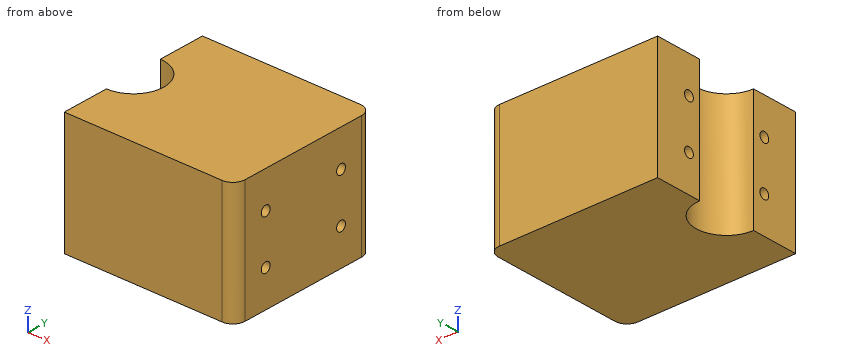
from build123d import *

# Parameters (mm, degrees)
F1_DEPTH = 25.4
F3_D     = 2.0828


# Not quite as in the source:
# - a feature names something its author has since deleted; it is built from what else it names


with BuildPart() as f1:
    # F0 (on Top) → F1 (new body)
    with BuildSketch(Plane.XY):
        with BuildLine():
            Line((-17.78, -6.35), (-17.78, -16.29156))
            Line((-17.78, -16.29156), (15.24, -16.29156))
            ThreePointArc((15.24, -16.29156), (17.0360512242, -15.5476112242), (17.78, -13.75156))
            Line((17.78, -13.75156), (17.78, 13.75156))
            ThreePointArc((17.78, 13.75156), (17.0360512242, 15.5476112242), (15.24, 16.29156))
            Line((15.24, 16.29156), (-17.78, 16.29156))
            Line((-17.78, 16.29156), (-17.78, 6.35))
            ThreePointArc((-17.78, 6.35), (-11.43, 0), (-17.78, -6.35))
        make_face()
    extrude(amount=F1_DEPTH)

    # F3 (through all)
    with Locations(Plane.YZ.offset(17.78)):
        with Locations((-8.89, 17.78), (-8.89, 7.62), (8.89, 17.78), (8.89, 7.62)):
            Hole(F3_D / 2)


solid = f1.part
Geometry: final body of the model. Coordinates: model frame, mm. Coordinates: 2 decimals unless noted, no trailing zeros. Write each loop counter-clockwise with the first axis right and the second up, starting at its lowest first coordinate (ties: lowest second). Pieces come first, ordered by that corner, then holes. Notation, with made-up numbers: (-6, -7.5) - (28, -7.5) arc R22 cw to (28, 27.5) - close; hole circle Ø9 at (32.25, -17). An arc over 180 degrees is marked (long way). Return JSON: item names as keys, results as strings.
Item 1: Section query D-D (z = 23.5). Output: boundary loops of the cut face in (x, y), and give its area (3 significant figures).
Completed:
{"outline": "(-17.78, -16.29) - (15.24, -16.29) arc R2.54 ccw to (17.78, -13.75) - (17.78, 13.75) arc R2.54 ccw to (15.24, 16.29) - (-17.78, 16.29) - (-17.78, 6.35) arc R6.35 cw to (-17.78, -6.35) - close", "area": "1,090 mm2"}
Item 2: Line query: L1, parallel to Z at x = -5, y = -8.89; L2, parallel to Z at x = 10, y = -8; L3, parallel to Y at x = -13.5, z = 4.25. Output: solid intervals per line, ascending.
Completed:
{"L1": "z = 0 to 6.58, 8.66 to 16.74, 18.82 to 25.4", "L2": "z = 0 to 7.08, 8.16 to 17.24, 18.32 to 25.4", "L3": "y = -16.29 to -4.69, 4.69 to 16.29"}
Item 3: Section query A-A (z = 7.62). Output: boundary loops of the cut face in (x, y), and give its area (3 significant figures).
Completed:
{"outline": "(-17.78, -16.29) - (15.24, -16.29) arc R2.54 ccw to (17.78, -13.75) - (17.78, -9.93) - (-17.78, -9.93) - close; (-17.78, -7.85) - (17.78, -7.85) - (17.78, 7.85) - (-17.78, 7.85) - (-17.78, 6.35) arc R6.35 cw to (-17.78, -6.35) - close; (-17.78, 9.93) - (17.78, 9.93) - (17.78, 13.75) arc R2.54 ccw to (15.24, 16.29) - (-17.78, 16.29) - close", "area": "944 mm2"}
Item 4: Section query C-C (x = 10.5). Output: boundary loops of the cut face in (y, z), and give its area (3 significant figures).
Completed:
{"outline": "(-16.29, 0) - (16.29, 0) - (16.29, 25.4) - (-16.29, 25.4) - close; hole circle Ø2.08 at (-8.89, 7.62); hole circle Ø2.08 at (-8.89, 17.78); hole circle Ø2.08 at (8.89, 7.62); hole circle Ø2.08 at (8.89, 17.78)", "area": "814 mm2"}
Item 5: Pin query (flat end, axial travel): pin 1 Ø5 at (y, z) = (2, 8) entering from -X. Return the tip coordinate at first contact, or that it passes through.
Completed:
{"pin 1": "stops at x = -13.3"}
Item 6: Section query B-B (y = 8.89). Output: boundary loops of the cut face in (x, z), and give its area (3 significant figures).
Completed:
{"outline": "(-17.78, 0) - (17.78, 0) - (17.78, 6.58) - (-17.78, 6.58) - close; (-17.78, 8.66) - (17.78, 8.66) - (17.78, 16.74) - (-17.78, 16.74) - close; (-17.78, 18.82) - (17.78, 18.82) - (17.78, 25.4) - (-17.78, 25.4) - close", "area": "755 mm2"}
